from build123d import *

# Parameters (mm, degrees)
SKETCH1_W           = 60
SKETCH1_H           = 32
BOSS_EXTRUDE1_DEPTH = 35
FILLET1_R           = 7
SKETCH3_R           = 1.75
BOSS_EXTRUDE3_DEPTH = 5


with BuildPart() as part:
    # Sketch1 → Boss-Extrude1 (new body)
    with BuildSketch(Plane.XY):
        Rectangle(SKETCH1_W, SKETCH1_H)
    extrude(amount=BOSS_EXTRUDE1_DEPTH)

    # Fillet1
    fillet1_edges = [part.edges().sort_by_distance(p)[0] for p in [
        (-30, 0, 35),
        (-30, 0, 0),
    ]]
    fillet(fillet1_edges, radius=FILLET1_R)

    # Sketch3 → Boss-Extrude3 (add)
    with BuildSketch(Plane(origin=(-30, 46, 0), x_dir=(0, 1, 0), z_dir=(-1, 0, 0))):
        with Locations(Location((-32.5, -11.3, 0), (0, 0, 90))):
            Circle(SKETCH3_R)
        with Locations(Location((-32.5, -23.7, 0), (0, 0, 90))):
            Circle(SKETCH3_R)
    extrude(amount=BOSS_EXTRUDE3_DEPTH)


solid = part.part
CAD build for the part. Positions are in the model's coordinates, mm. A direction names the side the tool comes from. Round coordinates to 2 decimals unless told otherwise and drop trailing zeros. Loops run counter-clockwise (first coordinate to the right, second up) from the corner with the lowest first, then second, coordinate; pieces in that order, holes last. Notation, with made-up numbers: M 26,-24.75 L 82,-24.75 A27 cw 82,-0.75 Z; hole C 82.5,40 d4. An arc over 180 degrees is marked long. One line per question, with ' | ' between items. Start each with the question number.
Item 1: Cut at C-C, the plane x = -27. Write the cut outline in (y, z).
Item 2: Wall check: line 1 (X direction, y = 5, z = 11.5); line 2 (X direction, y = -11, z = 2); line 3 (Z direction, x = -27, y = 7). Give the ranges that are in metal, low to high.
Item 3: Which spindle directions (+Z, -Z, +X, -X, +Y, -Y) get a long thin tool onto all of the face, cutting with end or side? Do faces 1 (the cylindrical face through (-32.465, 12.974, 22.031)), 2 (the flat face through (3, 0, 0)). Say none if no direction does.
Item 4: Two-plate mould, pull along Z, no slides. Class faces 3 (the flat face through (3, 0, 35)), 4 (the cylindrical face through (-28, 0.2, 2.1)), 5 (the cylindrical face through (-32.47, 12.32, 12.59)), 6 (the flat face through (-35, 13, 11)): pulls with the +Z half, pulls with the -Z half, needs draft (parallel to the pull), parting line crosses it, or undercut.
Item 5: Cut at A-A, the plane z = 23.7. Write the cut outline in (x, y).
Item 6: Pin check, flat tip, straight feed: pin 1 Ø2 at (y, z) = (6, 18.5) entering from -X. Stop position of the tip, or through.
Item 7: Cut at B-B, the plane y = 13.5. Write the cut outline in (x, z), plus the area to 3 significant figures.
Item 8: Cut at D-D, the plane z = 17. Write the cut outline in (x, y), plus the area to 3 significant figures.
Responses:
1) outline: M -16,1.26 L 16,1.26 L 16,33.74 L -16,33.74 Z
2) line 1: x = -30 to 30 | line 2: x = -27.9 to 30 | line 3: z = 1.26 to 33.74
3) face 1: -X | face 2: -Z, +X, -X, +Y, -Y
4) face 3: pulls with the +Z half | face 4: pulls with the -Z half | face 5: undercut | face 6: needs draft
5) outline: M -35,11.75 L -30,11.75 L -30,-16 L 30,-16 L 30,16 L -30,16 L -30,15.25 L -35,15.25 Z
6) pin 1: stops at x = -30
7) outline: M -35,9.55 L -30,9.55 L -30,7 A7 ccw -23,0 L 30,0 L 30,35 L -23,35 A7 ccw -30,28 L -30,25.45 L -35,25.45 L -35,21.95 L -30,21.95 L -30,13.05 L -35,13.05 Z | area: 2,110 mm²
8) outline: M -30,-16 L 30,-16 L 30,16 L -30,16 Z | area: 1,920 mm²
